Part print with two shaded views. Sizes in mm from the minimum x, y, z corner. A direction names the side the tool comes from. Round coordinates to 2 decimals unless told otherwise and drop trailing zeros. Write each loop counter-clockwise with the first axis right and the second up, starting at its lowest first coordinate (ties: lowest second). Pieces come first, ordered by that corner, then holes. Notation, with made-up numbers: (0, 70.25) -> (19, 70.25) arc R17 ccw to (19, 99.25) -> close; hole circle Ø7 at (70.5, 23). An arc over 180 degrees is marked (long way). Return JSON: item names as keys, results as strings.
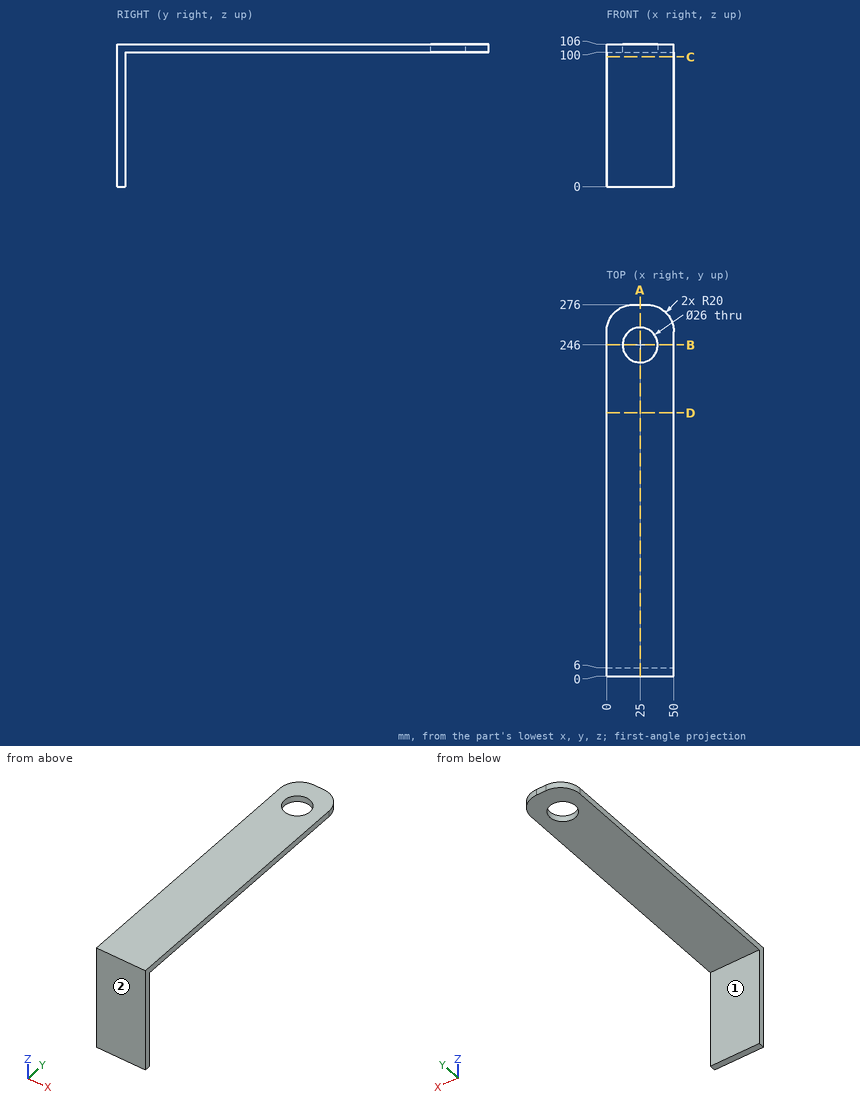
Q1. Saw through at B-B on y = 246. List the corners of the cut face in (x, z), then the cut area to 3 significant figures.
Verdict:
{"outline": "(0, 100) -> (12, 100) -> (12, 106) -> (0, 106) -> close; (38, 100) -> (50, 100) -> (50, 106) -> (38, 106) -> close", "area": "144 mm²"}
Q2. Saw through at D-D on y = 195.5. List the corners of the cut face in (x, z), then the cut area to 3 significant figures.
Verdict:
{"outline": "(0, 100) -> (50, 100) -> (50, 106) -> (0, 106) -> close", "area": "300 mm²"}
Q3. Saw through at C-C on z = 96.5. List the corners of the cut face in (x, y).
Verdict:
{"outline": "(0, 0) -> (50, 0) -> (50, 6) -> (0, 6) -> close"}
Q4. Pin check, flat tips, straight feed: pin 1 Ø12 at (x, y) = (14.5, 30) entering from -Z; pin 2 Ø10 at (x, z) = (31.5, 42) entering from +Y. Stop position of each tip, or through.
Verdict:
{"pin 1": "stops at z = 100", "pin 2": "stops at y = 6"}
Q5. Wall check: L1, parallel to Y at x = 25, z = 103; L2, parallel to Y at x = 43.5, z = 88; L3, parallel to Z at x = 46.5, y = 122.5. Give the ranges that are in metal, low to high.
Verdict:
{"L1": "y = 0 to 233, 259 to 276", "L2": "y = 0 to 6", "L3": "z = 100 to 106"}
Q6. 3-axis set-ups, long thin cutter, end or side, ignore diameter. For the marked faces 1 and 2: which of +Z, -Z, +X, -X, +Y, -Y reach the whole face in a straight line?
Verdict:
{"face 1": "-Z, +X, -X, +Y", "face 2": "+Z, -Z, +X, -X, -Y"}
Q7. Saw through at A-A on x = 25. List the corners of the cut face in (y, z).
Verdict:
{"outline": "(0, 0) -> (6, 0) -> (6, 100) -> (233, 100) -> (233, 106) -> (0, 106) -> close; (259, 100) -> (276, 100) -> (276, 106) -> (259, 106) -> close"}
